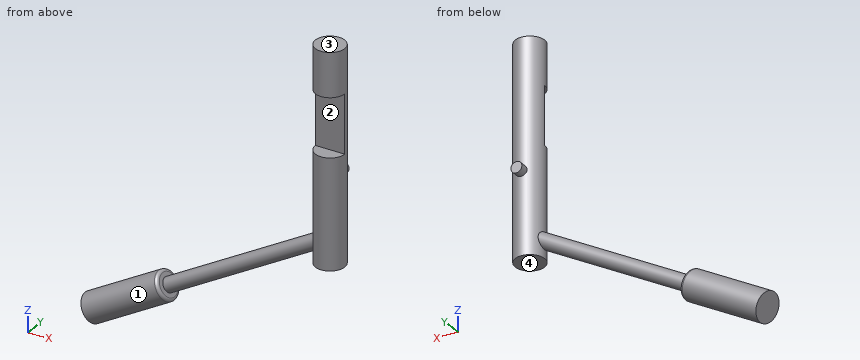
Solid Edge part; units mm, degrees
sketch "Sketch1" plane through (0, 0, 0) normal (0, 0, 1) x (1, 0, 0)
  circle A0 centre (0, 0) radius 2
extrude "Protrusion1" add sketch "Sketch1" along normal blind 29
sketch "Sketch2" plane through (-38.4939, 0, -4.7907) normal (-0.866, 0, -0.5) x (0.5, 0, -0.866)
  circle A0 centre (12.0981, 0) radius 1
extrude "Protrusion2" add sketch "Sketch2" against normal up to next
sketch "Sketch3" plane through (-38.4939, 0, -4.7907) normal (-0.866, 0, -0.5) x (0.5, 0, -0.866)
  circle A0 centre (12.0981, 0) radius 2
extrude "Top___Lever" add sketch "Sketch3" against normal blind 12
fillet "Round___Lever" radius 0.4 1 edges at (-23.0526, 0, -7.5359)
sketch "Sketch4" plane through (-2, 0, 14.5) normal (-1, 0, 0) x (0, 0, -1)
  line L0 (-0.5, 2) -> (-8.5, 2)
  line L1 (-8.5, 2) -> (-8.5, 0)
  line L2 (-8.5, 0) -> (-0.5, 0)
  line L3 (-0.5, 0) -> (-0.5, 2)
  dimension "D1" = 8.5
extrude "Cutout1" cut sketch "Sketch4" against normal up to next
sketch "Sketch5" plane through (0, 3, 14.5) normal (0, 1, 0) x (0, 0, -1)
  circle A0 centre (3.215, 0) radius 0.75
extrude "Protrusion3" add sketch "Sketch5" against normal up to next
properties material "ABS Plastic, high impact"
Here's how the part is built. I have some questions about the finished solid (model axes, mm). Face numbers are marked on the shaded views. Round coordinates to 2 decimals unless told otherwise and drop trailing zeros. Loops run counter-clockwise (first coordinate to the right, second up) from the corner with the lowest first, then second, coordinate; pieces in that order, holes last. Notation, with made-up numbers: (61.25, 21) -> (77.25, 21) arc R12 ccw to (77.25, 38) -> close; hole circle Ø8 at (27.5, -36.5). An arc over 180 degrees is marked (long way). Answer as CSV lines item,"result".
1. For pin 1 (1.6 mm diameter, centred on x = 1, y = -1, fed in from -Z); pin 2 (6 mm diameter, centred on x = -7, z = 18, fed in from -Y); pin 3 (3 mm diameter, centred on x = -27.5, y = 1.5, fed in from +Z); pin 4 (1.2 mm diameter, centred on x = -0.5, z = 19, fed in from -Y), each with a flat end and sliding along its axis, tell me the tip position at first contact or that it passes through.
Final values:
pin 1,"stops at z = 0"
pin 2,"passes through"
pin 3,"stops at z = -9.52"
pin 4,"stops at y = 0"
2. If we section it at C-C on z = 24.5: Please give me the cut outline in (x, y), plus the area to 3 significant figures.
Final values:
outline,"circle Ø4 at (0, 0)"
area,"12.6 mm^2"
3. If we section it at B-B on z = 16.5: Please give me the cut outline in (x, y).
Final values:
outline,"(-2, 0) -> (2, 0) arc R2 ccw to start"
4. If I drill on L1, parallel to Y at x = -27.5, z = -12.5; L2, parallel to Z at x = -16.5, y = 0.4, over which ranges is the centre line in solid material (lowest first)?
Final values:
L1,"y = -2 to 2"
L2,"z = -7.12 to -5"
5. Thinking about a two-plate mould opening in Z: for the marked faces 1, 2, 3 and 4, which applies, released by +Z, released by -Z, zero draft, split by the parting line, or undercut?
Final values:
face 1,"split by the parting line"
face 2,"undercut"
face 3,"released by +Z"
face 4,"released by -Z"
6. If we section it at A-A on x = 0: Please give me the cut outline in (y, z) (3 decimals).
Final values:
outline,"(-2, 0) -> (2, 0) -> (2, 10.535) -> (3, 10.535) -> (3, 12.035) -> (2, 12.035) -> (2, 29) -> (-2, 29) -> (-2, 23) -> (0, 23) -> (0, 15) -> (-2, 15) -> close"
